Can you work these out from the model? Positions are in its coordinate system, mm. A direction names the side the tool comes from. Coordinates: 2 decimals unless noted, no trailing zeros. Write each loop counter-clockwise with the first axis right and the second up, starting at its lowest first coordinate (ties: lowest second). Pieces come first, ordered by that corner, then holes. Notation, with made-up numbers: (69, 49) -> (125, 49) arc R23 cw to (125, 74) -> close; hole circle Ø2 at (-12.75, 88). An arc over 180 degrees is marked (long way). Use one line per item in the form item = value.
```python
from build123d import *

# Parameters (mm, degrees)
SKETCH_1_W                  = 15
SKETCH_1_H                  = 252
EXTRUDE_1_DEPTH             = 15
EXTRUDE_2_DEPTH             = 6
SKETCH_3_W                  = 8
SKETCH_3_H                  = 225
CUT_EXTRUDE_1_DEPTH         = 253.891280988
SKETCH_7_W                  = 15
SKETCH_7_H                  = 6
CUT_EXTRUDE_4_DEPTH         = 245.863737617
SKETCH_5_W                  = 8
SKETCH_5_H                  = 225
EXTRUDE_3_DEPTH             = 3
CUT_EXTRUDE_3_DEPTH         = 8
FILLET_1_R                  = 5
CHAMFER_1_SIZE              = 0.5
HOLE_WIZARD_M31_D           = 2.5
HOLE_WIZARD_M31_DEPTH       = 8.5
HOLE_WIZARD_M31_CSINK_D     = 3.05
HOLE_WIZARD_M31_CSINK_ANGLE = 120
HOLE_WIZARD_M31_TIP         = 0.751075774
HOLE_WIZARD_M41_D           = 4.5
HOLE_WIZARD_M41_CBORE_D     = 8
HOLE_WIZARD_M41_CBORE_DEPTH = 4.4
SKETCH_12_R                 = 3
CUT_EXTRUDE_5_DEPTH         = 5
CHAMFER_2_SIZE              = 1
HOLE_WIZARD_M21_D           = 1.6
HOLE_WIZARD_M21_DEPTH       = 6
HOLE_WIZARD_M21_CSINK_D     = 2.05
HOLE_WIZARD_M21_CSINK_ANGLE = 120
HOLE_WIZARD_M21_TIP         = 0.480688495


with BuildPart() as part:
    # Эскиз1 → Бобышка-Вытянуть1 (new body)
    with BuildSketch(Plane.XY):
        with Locations((7.5, 126)):
            Rectangle(SKETCH_1_W, SKETCH_1_H)
    extrude(amount=EXTRUDE_1_DEPTH)

    # Эскиз2 → Бобышка-Вытянуть2 (add)
    with BuildSketch(Plane.XY.offset(15)):
        Polygon((15, 8.5), (15, 243.5), (0, 243.5), (0, 238.5), (8, 238.5), (8, 13.5), (0, 13.5), (0, 8.5), align=None)
    extrude(amount=EXTRUDE_2_DEPTH)

    # Эскиз3 → Вырез-Вытянуть1 (cut, through all)
    with BuildSketch(Plane.XY.offset(15)):
        with Locations((4, 126)):
            Rectangle(SKETCH_3_W, SKETCH_3_H)
    extrude(amount=-CUT_EXTRUDE_1_DEPTH, mode=Mode.SUBTRACT)

    # Эскиз7 → Вырез-Вытянуть4 (cut, through all)
    with BuildSketch(Plane(origin=(0, 243.5, 0), x_dir=(1, 0, 0), z_dir=(0, 1, 0))):
        with Locations((7.5, -18)):
            Rectangle(SKETCH_7_W, SKETCH_7_H)
    extrude(amount=-CUT_EXTRUDE_4_DEPTH, mode=Mode.SUBTRACT)

    # Эскиз5 → Бобышка-Вытянуть3 (add)
    with BuildSketch(Plane.XY.offset(15)):
        with Locations((4, 126)):
            Rectangle(SKETCH_5_W, SKETCH_5_H)
    extrude(amount=-EXTRUDE_3_DEPTH)

    # Эскиз6 → Вырез-Вытянуть3 (cut)
    with BuildSketch(Plane.XY.offset(15)):
        with BuildLine():
            Line((8, 232), (8, 20))
            ThreePointArc((8, 20), (7, 19), (6, 20))
            Line((6, 20), (6, 232))
            ThreePointArc((6, 232), (7, 233), (8, 232))
        make_face()
    extrude(amount=-CUT_EXTRUDE_3_DEPTH, mode=Mode.SUBTRACT)

    # Скругление1
    fillet_1_edges = [part.edges().sort_by_distance(p)[0] for p in [
        (4, 238.5, 12),
        (4, 13.5, 12),
    ]]
    fillet(fillet_1_edges, radius=FILLET_1_R)

    # Фаска1
    chamfer_1_edges = [part.edges().sort_by_distance(p)[0] for p in [
        (15, 126, 15),
    ]]
    chamfer(chamfer_1_edges, length=CHAMFER_1_SIZE)

    # Отверстие обработанное метчиком M31
    with Locations(Plane.XY.offset(15)):
        with Locations((9, 5), (9, 247)):
            CounterSinkHole(HOLE_WIZARD_M31_D / 2, HOLE_WIZARD_M31_CSINK_D / 2, depth=HOLE_WIZARD_M31_DEPTH, counter_sink_angle=HOLE_WIZARD_M31_CSINK_ANGLE)
            with Locations((0, 0, -(HOLE_WIZARD_M31_DEPTH + HOLE_WIZARD_M31_TIP / 2))):  # 118° drill point
                Cone(0, HOLE_WIZARD_M31_D / 2, HOLE_WIZARD_M31_TIP, mode=Mode.SUBTRACT)

    # Цековка для  винта с внутренним шестигранником M41 (through all)
    with Locations(Plane(origin=(15, 0, 0), x_dir=(0, 0, -1), z_dir=(1, 0, 0))):
        with Locations((-8, 10), (-8, 242)):
            CounterBoreHole(HOLE_WIZARD_M41_D / 2, HOLE_WIZARD_M41_CBORE_D / 2, HOLE_WIZARD_M41_CBORE_DEPTH)

    # Эскиз12 → Вырез-Вытянуть5 (cut)
    with BuildSketch(Plane(origin=(15, 0, 0), x_dir=(0, 0, -1), z_dir=(1, 0, 0))):
        with Locations((-10, 232)):
            Circle(SKETCH_12_R)
        with Locations((-10, 20)):
            Circle(SKETCH_12_R)
    extrude(amount=-CUT_EXTRUDE_5_DEPTH, mode=Mode.SUBTRACT)

    # Фаска2
    chamfer_2_edges = [part.edges().sort_by_distance(p)[0] for p in [
        (8, 126, 0),
    ]]
    chamfer(chamfer_2_edges, length=CHAMFER_2_SIZE)

    # Отверстие обработанное метчиком M21
    with Locations(Plane(origin=(0, 0, 0), x_dir=(-1, 0, 0), z_dir=(0, 0, -1))):
        with Locations((-12, 101), (-12, 201), (-12, 151), (-12, 51)):
            CounterSinkHole(HOLE_WIZARD_M21_D / 2, HOLE_WIZARD_M21_CSINK_D / 2, depth=HOLE_WIZARD_M21_DEPTH, counter_sink_angle=HOLE_WIZARD_M21_CSINK_ANGLE)
            with Locations((0, 0, -(HOLE_WIZARD_M21_DEPTH + HOLE_WIZARD_M21_TIP / 2))):  # 118° drill point
                Cone(0, HOLE_WIZARD_M21_D / 2, HOLE_WIZARD_M21_TIP, mode=Mode.SUBTRACT)


solid = part.part
```
Q1. Suppose I cut it at A-A (y = 69.5). Write out the boundary of the cut face in (x, z), then the cut area to 3 significant figures.
Return value:
outline = (0, 12) -> (6, 12) -> (6, 15) -> (0, 15) -> close; (8, 1) -> (9, 0) -> (15, 0) -> (15, 14.5) -> (14.5, 15) -> (8, 15) -> close
area = 122 mm2
Q2. Suppose I cut it at B-B (x = 2.5). Write out the boundary of the cut face in (y, z).
Return value:
outline = (0, 0) -> (13.5, 0) -> (13.5, 7) arc R5 cw to (18.5, 12) -> (233.5, 12) arc R5 cw to (238.5, 7) -> (238.5, 0) -> (252, 0) -> (252, 15) -> (0, 15) -> close; hole circle Ø4.5 at (10, 8); hole circle Ø4.5 at (242, 8)
Q3. If I drill on line 1 (X direction, y = 103.5, z = 14); line 2 (Y direction, x = 11.75, z = 2.75); line 3 (Y direction, x = 7, z = 14.5), over which ranges is the centre line in solid material (lowest first)? Write a range as from..to.
Return value:
line_1 = 0..6, 8..15
line_2 = 0..50.24, 51.76..100.24, 101.76..150.24, 151.76..200.24, 201.76..252
line_3 = 0..19, 233..252
Q4. For faces 1 (the flat face through (4, 238.5, 4)), 2 (the flat face through (10.6, 8, 6)), 3 (the cylindrical face through (5.23, 244.23, 7.71)), which set-ups out of +Z, -Z, +X, -X, +Y, -Y let a thin tool reach every point of the face, with its end or its side?
Return value:
face_1 = -Z, -X
face_2 = +X
face_3 = +X, -X
Q5. Thinking about a two-plate mould opening in Y: for faces 4 (the cylindrical face through (12.5, 18.2, 12.4)), 5 (the flat face through (7, 0, 7)), 6 (the flat face through (15, 124, 7)), which applies, released by +Y, released by -Y, zero draft, split by the parting line, or undercut?
Return value:
face_4 = undercut
face_5 = released by -Y
face_6 = zero draft
Q6. Will these pins go through, and if not, where does the flat tip stop? pin 1 (2.5 mm diameter, centred on x = 3, y = 161, fed in from -Z); pin 2 (6.5 mm diameter, centred on y = 10, z = 8, fed in from +X); pin 3 (6 mm diameter, centred on x = 5.5, y = 180.5, fed in from -Z).
Return value:
pin_1 = 12
pin_2 = 10.6
pin_3 = 0.5
Q7. Suppose I cut it at C-C (y = 242). Write out the boundary of the cut face in (x, z).
Return value:
outline = (0, 0) -> (15, 0) -> (15, 4) -> (10.6, 4) -> (10.6, 5.75) -> (0, 5.75) -> close; (0, 10.25) -> (10.6, 10.25) -> (10.6, 12) -> (15, 12) -> (15, 14.5) -> (14.5, 15) -> (0, 15) -> close
